Read the model definition and answer for the solid it produces. Units are mm, in the model's axes. Face numbers are marked on the shaded views. A direction names the side the tool comes from. Coordinates: 2 decimals unless noted, no trailing zeros. Write each loop counter-clockwise with the first axis right and the second up, starting at its lowest first coordinate (ties: lowest second). Pieces come first, ordered by that corner, then holes. Notation, with made-up numbers: (46, 66.5) - (83, 66.5) arc R35 ccw to (83, 101.5) - close; hole circle Ø11 at (-22.5, -28). An arc over 180 degrees is marked (long way). Return JSON: item names as keys, results as strings.
```python
from build123d import *

# Parameters (mm, degrees)
SKETCH1_W                = 180
SKETCH1_H                = 34
BOSS_EXTRUDE1_DEPTH      = 50
FILLET1_R                = 10
CHAMFER1_SIZE            = 3
SKETCH2_R                = 28
BOSS_EXTRUDE2_DEPTH      = 20
SKETCH3_R                = 17.25
CUT_EXTRUDE1_DEPTH       = 117.258333035
SKETCH4_R                = 4
CUT_EXTRUDE2_DEPTH       = 109.425089347
FILLET2_R                = 2
F_6_0_6_DIAMETER_HOLE1_D = 6
CUT_EXTRUDE3_DEPTH       = 110.402925007
CUT_EXTRUDE3_DEPTH_BACK  = 110.402925007
SKETCH8_R                = 3


with BuildPart() as part:
    # Sketch1 → Boss-Extrude1 (new, symmetric)
    with BuildSketch(Plane.XY):
        Rectangle(SKETCH1_W, SKETCH1_H)
    extrude(amount=BOSS_EXTRUDE1_DEPTH, both=True)

    # Fillet1
    fillet1_edges = [part.edges().sort_by_distance(p)[0] for p in [
        (90, 0, 50),
        (-90, 0, 50),
        (90, 0, -50),
        (-90, 0, -50),
    ]]
    fillet(fillet1_edges, radius=FILLET1_R)

    # Chamfer1
    chamfer1_edges = [part.edges().sort_by_distance(p)[0] for p in [
        (0, -17, 50),
        (0, 17, 50),
        (0, -17, -50),
        (90, -17, 0),
        (-90, -17, 0),
        (87.071067812, -17, 47.071067812),
        (87.071067812, -17, -47.071067812),
        (-87.071067812, -17, -47.071067812),
        (-87.071067812, -17, 47.071067812),
        (-90, 17, 0),
        (0, 17, -50),
        (90, 17, 0),
        (87.071067812, 17, 47.071067812),
        (87.071067812, 17, -47.071067812),
        (-87.071067812, 17, -47.071067812),
        (-87.071067812, 17, 47.071067812),
    ]]
    chamfer(chamfer1_edges, length=CHAMFER1_SIZE)

    # Sketch2 → Boss-Extrude2 (add)
    with BuildSketch(Plane(origin=(0, 17, 0), x_dir=(1, 0, 0), z_dir=(0, 1, 0))):
        with Locations((-56, 0)):
            Circle(SKETCH2_R)
    extrude(amount=BOSS_EXTRUDE2_DEPTH)

    # Sketch3 → Cut-Extrude1 (cut, through all)
    with BuildSketch(Plane(origin=(0, 37, 0), x_dir=(1, 0, 0), z_dir=(0, 1, 0))):
        with Locations(Location((-56, 0, 0), (0, 0, 180))):
            Circle(SKETCH3_R)
    extrude(amount=-CUT_EXTRUDE1_DEPTH, mode=Mode.SUBTRACT)

    # Sketch4 → Cut-Extrude2 (cut, through all)
    with BuildSketch(Plane(origin=(0, 17, 0), x_dir=(1, 0, 0), z_dir=(0, 1, 0))):
        with Locations(Location((45, 0, 0), (0, 0, 180))):
            Circle(SKETCH4_R)
    extrude(amount=-CUT_EXTRUDE2_DEPTH, mode=Mode.SUBTRACT)

    # Fillet2
    fillet2_edges = [part.edges().sort_by_distance(p)[0] for p in [
        (-84, 17, 0),
    ]]
    fillet(fillet2_edges, radius=FILLET2_R)

    # Ø6.0 (6) Diameter Hole1 (through all)
    with Locations(Plane(origin=(0, 17, 0), x_dir=(1, 0, 0), z_dir=(0, 1, 0))):
        with Locations((80, -40), (-80, -40), (80, 40), (-80, 40)):
            Hole(F_6_0_6_DIAMETER_HOLE1_D / 2)

    # Sketch8 → Cut-Extrude3 (cut, two sides: drawn at the far end of the back side and taken through both)
    with BuildSketch(Plane.XY.offset(-CUT_EXTRUDE3_DEPTH_BACK)):
        with Locations((-56, 27)):
            Circle(SKETCH8_R)
    extrude(amount=CUT_EXTRUDE3_DEPTH + CUT_EXTRUDE3_DEPTH_BACK, mode=Mode.SUBTRACT)


solid = part.part
```
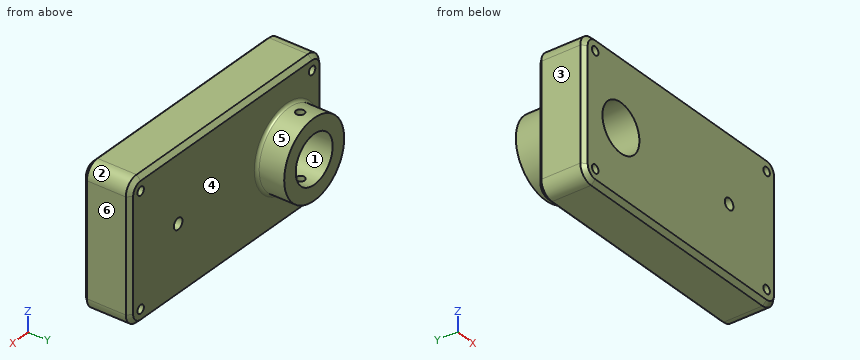
(1) Flat-ended cylindrical pins translate along their axes: P1, Ø9.5, axis at x = -56, y = 27, coming from the -Z side; P2, Ø5, axis at x = -80, z = -40, coming from the +Y side; P3, Ø3, axis at y = 23, z = -24, coming from the +X side; P4, Ø5, axis at y = 18.5, z = 11.5, coming from the -X side. Find the tip coordinate at first contact, or state that the pin passes through.
Answer:
{"P1": "z = -28", "P2": "through", "P3": "x = -39.33", "P4": "x = -88"}
(2) Determine the mould class of the marked faces 1, 2, 3 and 4 for opening direction X: +X half, -X half, draft (parallel to the pull), parting line (faces both ways), or undercut.
Answer:
{"face 1": "undercut", "face 2": "+X half", "face 3": "-X half", "face 4": "draft"}
(3) A cutting plane is placed at D-D (x = -56). Determine the outline of the cut face in (y, z).
Answer:
{"outline": "(-17, -47) - (-14, -50) - (14, -50) - (17, -47) - (17, -30) arc R2 cw to (19, -28) - (24, -28) - (24, -17.25) - (-17, -17.25) - close; (-17, 17.25) - (24, 17.25) - (24, 28) - (19, 28) arc R2 cw to (17, 30) - (17, 47) - (14, 50) - (-14, 50) - (-17, 47) - close; (30, -28) - (37, -28) - (37, -17.25) - (30, -17.25) - close; (30, 17.25) - (37, 17.25) - (37, 28) - (30, 28) - close"}
(4) A cutting plane is placed at B-B (y = 7.5). Determine the outline of the cut face in (x, z).
Answer:
{"outline": "(-90, -40) arc R10 ccw to (-80, -50) - (80, -50) arc R10 ccw to (90, -40) - (90, 40) arc R10 ccw to (80, 50) - (-80, 50) arc R10 ccw to (-90, 40) - close; hole circle Ø6 at (-80, -40); hole circle Ø6 at (-80, 40); hole circle Ø34.5 at (-56, 0); hole circle Ø8 at (45, 0); hole circle Ø6 at (80, -40); hole circle Ø6 at (80, 40)"}
(5) A cutting plane is placed at A-A (x = 45). Determine the outline of the cut face in (y, z).
Answer:
{"outline": "(-17, -47) - (-14, -50) - (14, -50) - (17, -47) - (17, -4) - (-17, -4) - close; (-17, 4) - (17, 4) - (17, 47) - (14, 50) - (-14, 50) - (-17, 47) - close"}
(6) Straight lines are drawn through the part: line 1 (Z direction, x = -80, y = -2.5); line 2 (X direction, y = 4, z = 40); line 3 (Y direction, x = -56.5, z = 26.5). For each, find the intervals that lie inside material, in ascending order. Write a range as from..to.
Answer:
{"line 1": "-50..-43, -37..37, 43..50", "line 2": "-90..-83, -77..77, 83..90", "line 3": "-17..24.04, 29.96..37"}
(7) A cutting plane is placed at C-C (z = 0). Determine the outline of the cut face in (x, y), and give its area (3 significant figures).
Answer:
{"outline": "(-90, -14) - (-87, -17) - (-73.25, -17) - (-73.25, 37) - (-84, 37) - (-84, 19) arc R2 cw to (-86, 17) - (-87, 17) - (-90, 14) - close; (-38.75, -17) - (41, -17) - (41, 17) - (-26, 17) arc R2 cw to (-28, 19) - (-28, 37) - (-38.75, 37) - close; (49, -17) - (87, -17) - (90, -14) - (90, 14) - (87, 17) - (49, 17) - close", "area": "5,090 mm²"}
(8) Which of the six approach directions +Z, -Z, +X, -X, +Y, -Y give full straight-line access (tool end or side, diameter ignored) to the marked faces 5 and 6?
Answer:
{"face 5": "+Y", "face 6": "+Z, -Z, +X, +Y, -Y"}
